Geometry check sheet. Reference: drawing and pictorial views, mm from the part's lowest x, y, z. A direction names the side the tool comes from. Give positions to 0.01 mm unless a question says otherwise; leave off trailing zeros. Order: outer loops, then holes, each group sorted by start corner. A loop starts at its lowest first (then second) coordinate and runs counter-clockwise, first axis right, second up. Notation, with made-up numbers: (15, 61) -> (50, 61) arc R3 ccw to (50, 65) -> close; hole circle Ø4 at (83, 30.25). An arc over 180 degrees is marked (long way). Write each question's results on one line, items separated by ' | '. Start each with the question number.
1. Cross-section at D-D, the plane z = 21. Enter the section's corners in (x, y), then the cut area to 3 significant figures.
2. Cross-section at B-B, the plane x = 12.5. Enter the section's corners in (y, z).
3. Cross-section at A-A, the plane y = 12.5. Enter the section's corners in (x, z), then the cut area to 3 significant figures.
4. Material ranges on L1, parallel to Z at x = 12.5, y = 17.75; L2, parallel to Z at x = 15.5, y = 13.25; L3, parallel to Z at x = 21, y = 7.5, recorded low to high. Write a range as from..to.
5. Depth check by flat-ended pin: pin 1 Ø8 at (x, y) = (21.5, 3.5) entering from -Z; pin 2 Ø1 at (x, z) = (4.5, 118.5) entering from +Y; pin 3 Ø2 at (x, z) = (16, 132) entering from -Y; pin 4 Ø8 at (x, z) = (12.5, 130.45) entering from -Y. Enter the tip coordinate at first touch or a pass-through.
6. Set-up check for the marked faces 1 and 2: record each of +Z, -Z, +X, -X, +Y, -Y from which the full face is reachable in a straight line by a thin tool's end or side.
7. Cross-section at C-C, the plane x = 20.25. Enter the section's corners in (y, z), then the cut area to 3 significant figures.
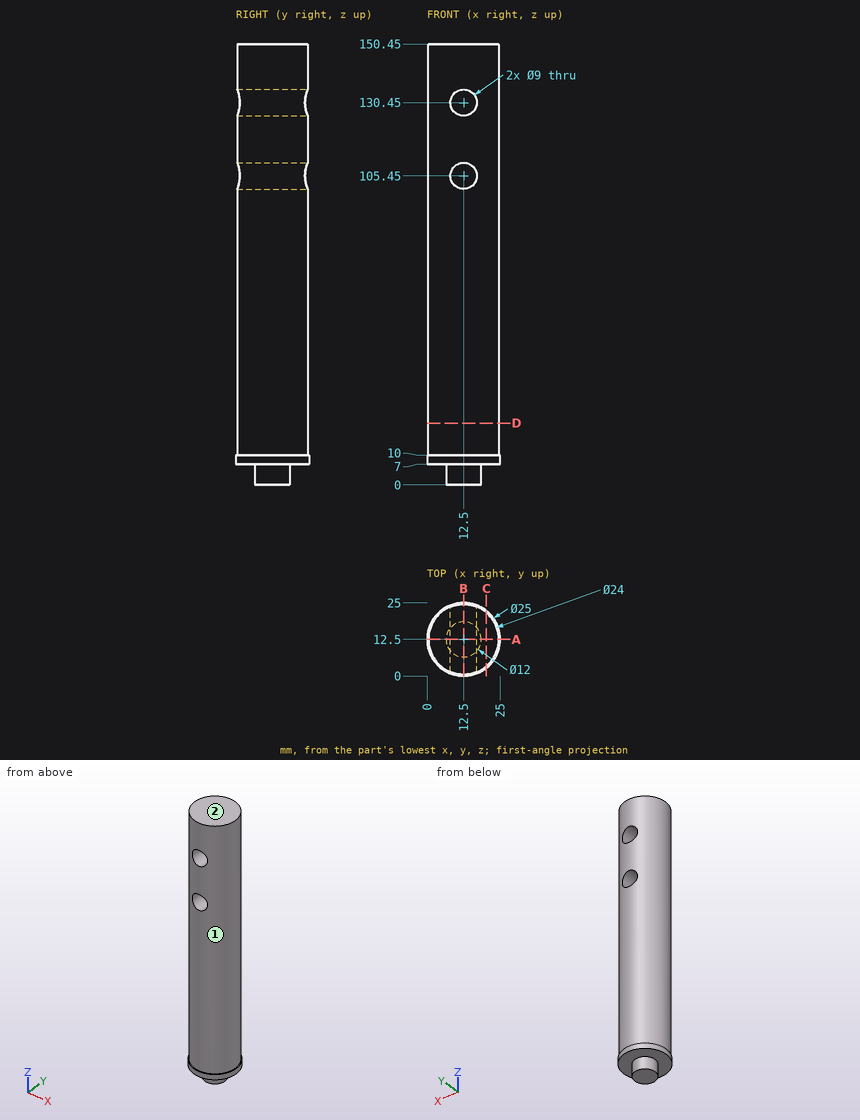
Results below:
1) outline: circle Ø24 at (12.5, 12.5) | area: 452 mm²
2) outline: (0, 7) -> (6.5, 7) -> (6.5, 0) -> (18.5, 0) -> (18.5, 7) -> (25, 7) -> (25, 10) -> (24.5, 10) -> (24.5, 100.95) -> (0.5, 100.95) -> (0.5, 10) -> (0, 10) -> close; (0.5, 109.95) -> (24.5, 109.95) -> (24.5, 125.95) -> (0.5, 125.95) -> close; (0.5, 134.95) -> (24.5, 134.95) -> (24.5, 150.45) -> (0.5, 150.45) -> close
3) outline: (0, 7) -> (6.5, 7) -> (6.5, 0) -> (18.5, 0) -> (18.5, 7) -> (25, 7) -> (25, 10) -> (24.5, 10) -> (24.5, 150.45) -> (0.5, 150.45) -> (0.5, 10) -> (0, 10) -> close; hole circle Ø9 at (12.5, 105.45); hole circle Ø9 at (12.5, 130.45) | area: 3,400 mm²
4) L1: z = 0..100.95, 109.95..125.95, 134.95..150.45 | L2: z = 0..102.1, 108.8..127.1, 133.8..150.45 | L3: z = 7..150.45
5) pin 1: stops at z = 7 | pin 2: stops at y = 21.87 | pin 3: stops at y = 1.09 | pin 4: passes through
6) face 1: +Z | face 2: +Z, +X, -X, +Y, -Y
7) outline: (2.69, 7) -> (22.31, 7) -> (22.31, 10) -> (21.66, 10) -> (21.66, 150.45) -> (3.34, 150.45) -> (3.34, 10) -> (2.69, 10) -> close | area: 2,630 mm²
